Part model, mm, in its own coordinate system. Give positions to 0.01 mm unless a question says otherwise; leave off trailing zeros. Order: outer loops, then holes, each group sorted by start corner. A loop starts at its lowest first (then second) coordinate and runs counter-clockwise, first axis right, second up.
1. Mould opens along X. For faces 1 (the cylindrical face through (-18.812, -79.922, 2.325)), 2 (the cylindrical face through (0.488, 90.166, 1.565)) say: +X half, -X half, draft (parallel to the pull), parting line (faces both ways), or undercut.
2. Probe line 1 (X direction, y = -34, z = 0.75) (3 decimals); line 2 (X direction, y = 27, z = 1.1) (3 decimals). List the from-to ranges inside material, lowest first.
3. Slice it at C-C on x = 12. List the corners of the cut face in (y, z) (1 decimal), and give its area (3 significant figures).
4. Drop a flat-ended pin along its axis: pin 1 Ø4 at (x, y) = (17.46, 92.36) entering from -Z. Give the stop position or say it passes through.
5. Slice it at B-B on z = 2.3. Give the number of separate pieces and of enclosed holes in the cut face, and give its area (3 significant figures).
6. Slice it at A-A on x = -11.5. List the corners of the cut face in (y, z) (1 decimal).
from build123d import *

# Parameters (mm, degrees)
SKETCH1_W                                       = 56.55
SKETCH1_H                                       = 197.425
BOSS_EXTRUDE1_DEPTH                             = 3.175
SKETCH2_R                                       = 5
CUT_EXTRUDE1_DEPTH                              = 103.731270343
SKETCH5_W                                       = 3.175
SKETCH5_H                                       = 197.425
BOSS_EXTRUDE2_DEPTH                             = 19.525
SKETCH14_W                                      = 76.075
SKETCH14_H                                      = 3.175
BOSS_EXTRUDE3_DEPTH                             = 3.175
M4_CLEARANCE_HOLE1_D                            = 4.5
CSK_FOR_M3_FLAT_HEAD_MACHINE_SCREW3_D           = 3.4
CSK_FOR_M3_FLAT_HEAD_MACHINE_SCREW3_CSINK_D     = 6.3
CSK_FOR_M3_FLAT_HEAD_MACHINE_SCREW3_CSINK_ANGLE = 90


with BuildPart() as part:
    # Sketch1 → Boss-Extrude1 (new body)
    with BuildSketch(Plane.XY):
        Rectangle(SKETCH1_W, SKETCH1_H)
    extrude(amount=BOSS_EXTRUDE1_DEPTH)

    # Sketch2 → Cut-Extrude1 (cut, through all)
    with BuildSketch(Plane(origin=(0, 0, 0), x_dir=(-1, 0, 0), z_dir=(0, 0, -1))):
        with Locations((-11.5, 30.630837161)):
            Circle(SKETCH2_R)
        with Locations((-11.5, 52.630837161)):
            Circle(SKETCH2_R)
        with Locations((-11.5, 41.630837161)):
            Circle(SKETCH2_R)
        with Locations((0, 52.630837161)):
            Circle(SKETCH2_R)
        with Locations((0, 41.630837161)):
            Circle(SKETCH2_R)
        with Locations((0, 30.630837161)):
            Circle(SKETCH2_R)
        with Locations((11.5, 30.630837161)):
            Circle(SKETCH2_R)
        with Locations((11.5, 41.630837161)):
            Circle(SKETCH2_R)
        with Locations((11.5, 52.630837161)):
            Circle(SKETCH2_R)
        with Locations((-11.5, -35.369162839)):
            Circle(SKETCH2_R)
        with Locations((-11.5, -13.369162839)):
            Circle(SKETCH2_R)
        with Locations((-11.5, -24.369162839)):
            Circle(SKETCH2_R)
        with Locations((0, -13.369162839)):
            Circle(SKETCH2_R)
        with Locations((0, -24.369162839)):
            Circle(SKETCH2_R)
        with Locations((0, -35.369162839)):
            Circle(SKETCH2_R)
        with Locations((11.5, -35.369162839)):
            Circle(SKETCH2_R)
        with Locations((11.5, -13.369162839)):
            Circle(SKETCH2_R)
        with Locations((11.5, -24.369162839)):
            Circle(SKETCH2_R)
    extrude(amount=-CUT_EXTRUDE1_DEPTH, mode=Mode.SUBTRACT)

    # Sketch5 → Boss-Extrude2 (add)
    with BuildSketch(Plane.ZY.offset(28.275)):
        with Locations((1.5875, 0)):
            Rectangle(SKETCH5_W, SKETCH5_H)
    extrude(amount=BOSS_EXTRUDE2_DEPTH)

    # Sketch14 → Boss-Extrude3 (add)
    with BuildSketch(Plane(origin=(0, 98.7125, 0), x_dir=(1, 0, 0), z_dir=(0, 1, 0))):
        with Locations((-9.7625, -1.5875)):
            Rectangle(SKETCH14_W, SKETCH14_H)
    extrude(amount=BOSS_EXTRUDE3_DEPTH)

    # M4 Clearance Hole1 (through all)
    with Locations(Plane.XY.offset(3.175)):
        with Locations((0, 92.3625001), (0, -78.8874999)):
            Hole(M4_CLEARANCE_HOLE1_D / 2)

    # CSK for M3 Flat Head Machine Screw3 (through all)
    with Locations(Plane(origin=(0, 0, 0), x_dir=(-1, 0, 0), z_dir=(0, 0, -1))):
        with Locations((17.4625, -78.8874999), (-17.4625, 92.3625001)):
            CounterSinkHole(CSK_FOR_M3_FLAT_HEAD_MACHINE_SCREW3_D / 2, CSK_FOR_M3_FLAT_HEAD_MACHINE_SCREW3_CSINK_D / 2, counter_sink_angle=CSK_FOR_M3_FLAT_HEAD_MACHINE_SCREW3_CSINK_ANGLE)


solid = part.part
Data:
1. face 1: undercut
1. face 2: undercut
2. line 1: x = -47.8 to -16.309, -6.691 to -4.809, 4.809 to 6.691, 16.309 to 28.275
2. line 2: x = -47.8 to -14.938, -8.062 to -3.438, 3.438 to 8.062, 14.938 to 28.275
3. outline: (-98.7, 0) - (-40.3, 0) - (-40.3, 3.2) - (-98.7, 3.2) - close; (-30.4, 0) - (-29.3, 0) - (-29.3, 3.2) - (-30.4, 3.2) - close; (-19.4, 0) - (-18.3, 0) - (-18.3, 3.2) - (-19.4, 3.2) - close; (-8.4, 0) - (25.7, 0) - (25.7, 3.2) - (-8.4, 3.2) - close; (35.6, 0) - (36.7, 0) - (36.7, 3.2) - (35.6, 3.2) - close; (46.6, 0) - (47.7, 0) - (47.7, 3.2) - (46.6, 3.2) - close; (57.6, 0) - (101.9, 0) - (101.9, 3.2) - (57.6, 3.2) - close
3. area: 447 mm2
4. pin 1: stops at z = 1.15
5. separate pieces: 1
5. enclosed holes: 22
5. area: 13,800 mm2
6. outline: (-98.7, 0) - (-40.4, 0) - (-40.4, 3.2) - (-98.7, 3.2) - close; (-30.4, 0) - (-29.4, 0) - (-29.4, 3.2) - (-30.4, 3.2) - close; (-19.4, 0) - (-18.4, 0) - (-18.4, 3.2) - (-19.4, 3.2) - close; (-8.4, 0) - (25.6, 0) - (25.6, 3.2) - (-8.4, 3.2) - close; (35.6, 0) - (36.6, 0) - (36.6, 3.2) - (35.6, 3.2) - close; (46.6, 0) - (47.6, 0) - (47.6, 3.2) - (46.6, 3.2) - close; (57.6, 0) - (101.9, 0) - (101.9, 3.2) - (57.6, 3.2) - close
